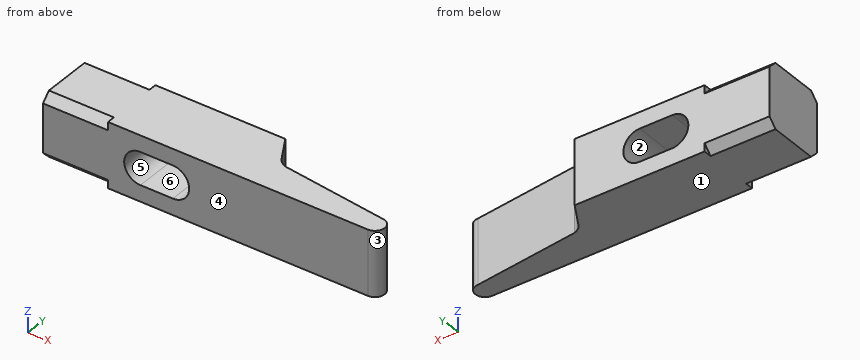
```python
from build123d import *

# Parameters (mm, degrees)
EXTRUDE_1_DEPTH     = 10
CUT_EXTRUDE_1_DEPTH = 106.399240984
CUT_EXTRUDE_2_DEPTH = 20


with BuildPart() as part:
    # 草图1 → 凸台-拉伸1 (new, symmetric)
    with BuildSketch(Plane.XY):
        with BuildLine():
            Line((0, 0), (0, 20))
            Line((0, 20), (60, 20))
            Line((60, 20), (64.330127019, 12.5))
            ThreePointArc((64.330127019, 12.5), (65.537347332, 11.095201195), (67.173135447, 10.226272076))
            Line((67.173135447, 10.226272076), (100, 6))
            ThreePointArc((100, 6), (103, 3), (100, 0))
            Line((100, 0), (0, 0))
        make_face()
    extrude(amount=EXTRUDE_1_DEPTH, both=True)

    # 草图2 → 切除-拉伸1 (cut, through all)
    with BuildSketch(Plane(origin=(0, 20, 0), x_dir=(1, 0, 0), z_dir=(0, 1, 0))):
        with BuildLine():
            Line((30, 5), (40, 5))
            ThreePointArc((40, 5), (45, 0), (40, -5))
            Line((40, -5), (30, -5))
            ThreePointArc((30, -5), (25, 0), (30, 5))
        make_face()
    extrude(amount=-CUT_EXTRUDE_1_DEPTH, mode=Mode.SUBTRACT)

    # 草图3 → 切除-拉伸2 (cut)
    with BuildSketch(Plane.ZY):
        Polygon((-10, 17.5), (-7.5, 20), (-10, 20), align=None)
        Polygon((10, 20), (7.5, 20), (10, 17.5), align=None)
        Polygon((10, 0), (10, 2.5), (7.5, 0), align=None)
        Polygon((-7.5, 0), (-10, 2.5), (-10, 0), align=None)
    extrude(amount=-CUT_EXTRUDE_2_DEPTH, mode=Mode.SUBTRACT)


solid = part.part
```
For this review, take the finished solid that the model builds, in its own axes (mm). Face numbers are marked on the shaded views. A direction names the side the tool comes from. Coordinates: 2 decimals unless noted, no trailing zeros. Loops run counter-clockwise (first coordinate to the right, second up) from the corner with the lowest first, then second, coordinate; pieces in that order, holes last. Notation, with made-up numbers: (48.5, -26.5) - (61.5, -26.5) arc R26 ccw to (61.5, 6.5) - close; hole circle Ø1 at (-12, -16.75). An arc over 180 degrees is marked (long way). Use one line per item in the form item = value. Start each with the question number.
1) For pin 1 (4 mm diameter, centred on y = 6, z = -1, fed in from +X); pin 2 (1 mm diameter, centred on x = 84, z = 3, fed in from +Y), all flat-tipped, find the tip position at first contact; note any pin that passes through.
2) Take a section at B-B (x = 37). State the section outline as (y, z) points, plus the area to 3 significant figures.
3) Draft analysis for pull direction X (two halves, no side actions). For the marked faces 3, 4, 5 and 6, state which applies: released by +X, released by -X, zero draft, split by the parting line, or undercut.
4) For the marked faces 1 and 2, list the 3-axis set-ups (+Z, -Z, +X, -X, +Y, -Y) from which the entire face can be reached by the end or side of a thin tool; tool diameter is ignored.
5) Take a section at D-D (x = 96). State the section outline as (y, z) points.
6) Take a section at C-C (y = 3.75). State the section outline as (x, z) points.
7) Take a section at A-A (z = 0). State the section outline as (x, y) points, plus the area to 3 significant figures.
8) To check wall thickness, follow probe 1 along Z at (x, y) = (35.5, 14); probe 2 along X at (y, z) = (12.75, 1.75); probe 3 along X at (y, z) = (16.75, -4). State the ranges of each line that lie inside material, in increasing order. Write a range as from..to.
From the geometry:
q1.pin_1 = 102.83
q1.pin_2 = 8.12
q2.outline = (0, -10) - (20, -10) - (20, -5) - (0, -5) - close; (0, 5) - (20, 5) - (20, 10) - (0, 10) - close
q2.area = 200 mm2
q3.face_3 = released by +X
q3.face_4 = zero draft
q3.face_5 = undercut
q3.face_6 = undercut
q4.face_1 = -Z, +X, -X, +Y, -Y
q4.face_2 = +Y, -Y
q5.outline = (0, -10) - (6.51, -10) - (6.51, 10) - (0, 10) - close
q6.outline = (0, -10) - (102.9, -10) - (102.9, 10) - (0, 10) - close; hole (30, -5) - (40, -5) arc R5 ccw to (40, 5) - (30, 5) arc R5 ccw to start
q7.outline = (0, 0) - (25, 0) - (25, 20) - (0, 20) - close; (45, 0) - (100, 0) arc R3 ccw to (100, 6) - (67.17, 10.23) arc R5 cw to (64.33, 12.5) - (60, 20) - (45, 20) - close
q7.area = 1,180 mm2
q8.probe_1 = -10..-5, 5..10
q8.probe_2 = 0..25.32, 44.68..64.19
q8.probe_3 = 0..27, 43..61.88
